The model under review builds one solid part; all positions refer to its coordinate system, in mm. A direction names the side the tool comes from. Coordinates: 2 decimals unless noted, no trailing zeros. Order: outer loops, then holes, each group sorted by start corner. A loop starts at its lowest first (then second) coordinate and runs counter-clockwise, first axis right, second up. Notation, with made-up numbers: (66.5, 69) -> (115.5, 69) arc R21 cw to (115.5, 95) -> close; hole circle Ø1 at (89.25, 16.25). An arc over 180 degrees is marked (long way). Use one line per item in the form item = value. Start each with the question number.
(1) Take a section at A-A (x = -21). State the section outline as (y, z) points.
(2) Insertion check: pin 1 Ø9.5 at (y, z) = (-5, -4) entering from +X; pin 2 Ø6 at (x, z) = (7, -4) entering from +Y; pin 3 Ø1.5 at (x, z) = (-10, 4.5) entering from +Y; pin 4 Ø10 at (x, z) = (16, 0.5) entering from -Y. Each pin has a flat end and moves straight along its axis. Give the tip position at first contact, or say it passes through.
(3) For faces 4 (the flat face through (-59.134, 0.2, -6.5)), 5 (the flat face through (-67.612, -3, 5)), 6 (the conical face through (-67.66, -9.88, 0.02)), list the 3-axis set-ups (+Z, -Z, +X, -X, +Y, -Y) from which the entire face can be reached by the end or side of a thin tool; tool diameter is ignored.
(4) Wall thickness on line 1 along X through (y, z) = (-7, 5.75); line 2 along Z through (x, y) = (-3.5, -0.25); line 3 along Z through (x, y) = (-21.5, -1.75): over which ranges is each line inside the solid? List them lowest first.
(5) Mouldability with a two-part tool opening along Z and no side actions: class faces 1 (the flat face through (-67.612, -3, -5)), 2 (the cylindrical face through (4.65, -6.2, 1.38)), 3 (the flat face through (-63.44, 8.21, 4.83)) as +Z half, -Z half, draft (parallel to the pull), parting line (faces both ways), or undercut.
```python
from build123d import *

# Parameters (mm, degrees)
SKETCH5_R           = 6.35
BOSS_EXTRUDE3_DEPTH = 127
CHAMFER1_SIZE       = 1.195753846
BOSS_EXTRUDE4_DEPTH = 8.73125
SKETCH8_OUTSIDE_W   = 522.464
SKETCH8_OUTSIDE_H   = 525.412
SKETCH8_OUTSIDE_R   = 9.525
CUT_EXTRUDE3_DEPTH  = 136.73125
CUT_EXTRUDE3_TAPER  = 60
CUT_EXTRUDE4_DEPTH  = 0.254
CIRPATTERN1_COUNT   = 3


with BuildPart() as part:
    # Sketch5 → Boss-Extrude3 (new body)
    with BuildSketch(Plane(origin=(67.865625, 0, 0), x_dir=(0, 0, -1), z_dir=(1, 0, 0))):
        Circle(SKETCH5_R)
    extrude(amount=-BOSS_EXTRUDE3_DEPTH)

    # Chamfer1
    chamfer1_edges = [part.edges().sort_by_distance(p)[0] for p in [
        (67.865625, 0, 6.35),
    ]]
    chamfer(chamfer1_edges, length=CHAMFER1_SIZE)

    # Sketch6 → Boss-Extrude4 (add)
    with BuildSketch(Plane.ZY.offset(59.134375)):
        Polygon((9.525, 5.499261314), (0, 10.998522628), (-9.525, 5.499261314), (-9.525, -5.499261314), (0, -10.998522628), (9.525, -5.499261314), align=None)
    extrude(amount=BOSS_EXTRUDE4_DEPTH)

    # Sketch8 outside → Cut-Extrude3 (cut, through all)
    with BuildSketch(Plane.ZY.offset(67.865625)):
        Rectangle(SKETCH8_OUTSIDE_W, SKETCH8_OUTSIDE_H)
        Circle(SKETCH8_OUTSIDE_R, mode=Mode.SUBTRACT)
    extrude(amount=-CUT_EXTRUDE3_DEPTH, taper=CUT_EXTRUDE3_TAPER, mode=Mode.SUBTRACT)

    # Sketch12 → Cut-Extrude4 (cut)
    with BuildSketch(Plane.ZY.offset(67.865625)):
        with BuildLine():
            Line((0.28575, 7.33425), (0.28575, 4.09575))
            ThreePointArc((0.28575, 4.09575), (0, 3.81), (-0.28575, 4.09575))
            Line((-0.28575, 4.09575), (-0.28575, 7.33425))
            ThreePointArc((-0.28575, 7.33425), (0, 7.62), (0.28575, 7.33425))
        make_face()
    cut_extrude4 = extrude(amount=-CUT_EXTRUDE4_DEPTH, mode=Mode.SUBTRACT)

    # CirPattern1: Cut-Extrude4 ×3 about axis
    cirpattern1_axis = Axis((0, 0, 0), (1, 0, 0))
    for i in range(1, CIRPATTERN1_COUNT):
        add(cut_extrude4.rotate(cirpattern1_axis, i * 360 / CIRPATTERN1_COUNT), mode=Mode.SUBTRACT)


solid = part.part
```
Findings:
q1.outline = circle Ø12.7 at (0, 0)
q2.pin_1 = 67.87
q2.pin_2 = 6.27
q2.pin_3 = 5.12
q2.pin_4 = -6.35
q3.face_4 = +X
q3.face_5 = -X
q3.face_6 = -X, -Y
q4.line_1 = -67.87 to -59.13
q4.line_2 = -6.35 to 6.35
q4.line_3 = -6.1 to 6.1
q5.face_1 = undercut
q5.face_2 = parting line
q5.face_3 = +Z half
